Autodesk Inventor part; units mm, degrees
ref_plane "YZ Plane" through (0, 0, 0) normal (1, 0, 0) x (0, 1, 0)
ref_plane "XZ Plane" through (0, 0, 0) normal (0, 1, 0) x (-1, 0, 0)
ref_plane "XY Plane" through (0, 0, 0) normal (0, 0, 1) x (1, 0, 0)
sketch "Sketch1" plane through (0, 0, 0) normal (0, 1, 0) x (-1, 0, 0)
  line L0 (0, 0) -> (25.4, 0)
  line L1 (25.4, 0) -> (25.4, -50.8)
  line L2 (25.4, -50.8) -> (0, -50.8)
  line L3 (0, -50.8) -> (0, 0)
  line L4 (22.225, -47.625) -> (22.225, -3.175)
  line L5 (22.225, -3.175) -> (3.175, -3.175)
  line L6 (3.175, -3.175) -> (3.175, -47.625)
  line L7 (3.175, -47.625) -> (22.225, -47.625)
  dimension "d0" = 50.8
  dimension "d1" = 25.4
  dimension "d2" = 3.175
extrude "Extrusion1" add sketch "Sketch1" along normal blind 406.4
sketch "Sketch2" plane through (0, 0, 0) normal (1, 0, 0) x (0, 0, -1)
  circle A0 centre (25.4, 203.2) radius 12.7
  line L0 (0, 0) -> (0, 406.4)
  line L1 (50.8, 0) -> (0, 0)
  dimension "d5" = 25.4
  dimension "d6" = 25.4
  dimension "d7" = 203.2
extrude "Extrusion2" cut sketch "Sketch2" against normal blind 25.4
sketch "Sketch4" plane through (-22.225, 0, -47.625) normal (1, 0, 0) x (0, 0, -1)
  circle A0 centre (-22.225, 320.675) radius 7.62
  line L0 (-47.625, 406.4) -> (3.175, 406.4)
  line L1 (-47.625, 0) -> (-47.625, 406.4)
  dimension "d15" = 25.4
  dimension "d16" = 15.24
  dimension "d25" = 85.725
extrude "Extrusion4" cut sketch "Sketch4" along normal blind 25.4
sketch "Sketch5" plane through (-22.225, 0, -47.625) normal (1, 0, 0) x (0, 0, -1)
  line L0 (0, 342.9) -> (-44.45, 342.9)
  line L1 (-44.45, 342.9) -> (-44.45, 298.45)
  line L2 (-44.45, 298.45) -> (0, 298.45)
  line L3 (0, 298.45) -> (0, 342.9)
  line L4 (0, 342.9) -> (0, 298.45)
  line L5 (-44.45, 298.45) -> (-44.45, 342.9)
  line L6 (0, 298.45) -> (-44.45, 298.45)
  line L7 (-44.45, 342.9) -> (0, 342.9)
  point P0 (-47.625, 0)
  dimension "d19" = 0
  dimension "d20" = 0
  dimension "d21" = 0
  dimension "d22" = 0
extrude "Extrusion5" cut sketch "Sketch5" against normal blind 25.4
properties part number "2x1 16in Aluminum-ver2-1111-2020"
For this review, take the finished solid that the model builds, in its own axes (mm). A direction names the side the tool comes from. Give positions to 0.01 mm unless a question says otherwise; leave off trailing zeros. Order: outer loops, then holes, each group sorted by start corner. A loop starts at its lowest first (then second) coordinate and runs counter-clockwise, first axis right, second up. Notation, with made-up numbers: (-22.5, -3.75) - (24.5, -3.75) arc R25 cw to (24.5, 8.25) - close; hole circle Ø8 at (-20, 75). An arc over 180 degrees is marked (long way). Answer as a JSON object with one key per item and string values. Group by question number.
Item 1: Clearance check with a flat-ended pin moving along its axis: pin 1 Ø20 at (y, z) = (320.675, -25.4) entering from -X (3 decimals). State where the tip first meets the part, or that it passes through.
Item 2: Take a section at C-C on x = -9. Give the boundary of the cut face in (y, z) (3 decimals), and give its area (3 significant figures).
Item 3: Draft analysis for pull direction Z (two halves, no side actions). For faces 1 (the flat face through (-13, 200, 0)), 2 (the flat face through (-2, 406.4, -27)), 3 (the flat face through (-14, 206, -3.175)), state which applies: pulls with the +Z half, pulls with the -Z half, needs draft (parallel to the pull), parting line crosses it, or undercut.
Item 4: Machinability: for faces 4 (the cylindrical face through (-23.79, 215.792, -23.747)), 5 (the flat face through (-22.225, 147, -26)), which of the approach directions +Z, -Z, +X, -X, +Y, -Y give a long, thin tool a straight path to every point of the face, cutting with its end or side? Answer none if there is none.
Item 5: Wall thickness on line 1 along Y through (x, z) = (-1.9, -25.4) (3 decimals); line 2 along X through (y, z) = (362.5, -12.5) (3 decimals); line 3 along Z through (x, y) = (-16, 18.5) (3 decimals): over which ranges is each line inside the solid? List them lowest first.
Item 6: Take a section at B-B on y = 183.5. Give the boundary of the cut face in (x, z) (3 decimals).
Item 7: Take a section at A-A on z = -25.4. Give the boundary of the cut face in (x, y) (3 decimals).
Item 8: Take a section at D-D on z = -7.5. Give the boundary of the cut face in (x, y) (3 decimals), and give its area (3 significant figures).
Reported:
{
 "1": {"pin 1": "x = -3.175"},
 "2": {"outline": "(0, -50.8) - (406.4, -50.8) - (406.4, -47.625) - (0, -47.625) - close; (0, -3.175) - (406.4, -3.175) - (406.4, 0) - (0, 0) - close", "area": "2,580 mm^2"},
 "3": {"face 1": "pulls with the +Z half", "face 2": "needs draft", "face 3": "undercut"},
 "4": {"face 4": "+X, -X", "face 5": "+Y, -Y"},
 "5": {"line 1": "0 to 190.5, 215.9 to 313.055, 328.295 to 406.4", "line 2": "-25.4 to -22.225, -3.175 to 0", "line 3": "-50.8 to -47.625, -3.175 to 0"},
 "6": {"outline": "(-25.4, -50.8) - (0, -50.8) - (0, 0) - (-25.4, 0) - close; hole (-22.225, -47.625) - (-3.175, -47.625) - (-3.175, -3.175) - (-22.225, -3.175) - close"},
 "7": {"outline": "(-25.4, 0) - (-22.225, 0) - (-22.225, 190.5) - (-25.4, 190.5) - close; (-25.4, 215.9) - (-22.225, 215.9) - (-22.225, 298.45) - (-25.4, 298.45) - close; (-25.4, 342.9) - (-22.225, 342.9) - (-22.225, 406.4) - (-25.4, 406.4) - close; (-3.175, 0) - (0, 0) - (0, 190.5) - (-3.175, 190.5) - close; (-3.175, 215.9) - (0, 215.9) - (0, 313.055) - (-3.175, 313.055) - close; (-3.175, 328.295) - (0, 328.295) - (0, 406.4) - (-3.175, 406.4) - close"},
 "8": {"outline": "(-25.4, 0) - (-22.225, 0) - (-22.225, 298.45) - (-25.4, 298.45) - close; (-25.4, 342.9) - (-22.225, 342.9) - (-22.225, 406.4) - (-25.4, 406.4) - close; (-3.175, 0) - (0, 0) - (0, 406.4) - (-3.175, 406.4) - close", "area": "2,440 mm^2"}
}
